Geometry check sheet. Reference: the model listing, model coordinates, mm. A direction names the side the tool comes from. Give positions to 0.01 mm unless a question says otherwise; leave off trailing zeros. Loops run counter-clockwise (first coordinate to the right, second up) from the corner with the lowest first, then second, coordinate; pieces in that order, holes last.
1. Go/stop test with flat-tipped pins: pin 1 Ø14 at (x, y) = (-53, 89.5) entering from -Z; pin 2 Ø1.2 at (y, z) = (77.5, 21) entering from +X. Record where each tip stops, or that it passes through.
2. Tool access check on faces 1 (the flat face through (-48, 0, 16)), 2 (the flat face through (-27, 63, 22.479)), 3 (the flat face through (-59, 63, 5.033)). Record the directions out of +Z, -Z, +X, -X, +Y, -Y that give a thin tool (end or side, any length) a straight path to the whole face; none if there is none.
3. Cross-section at B-B, the plane y = 29.5. Record the cut outline in (x, z), plus the area to 3 significant figures.
4. Cross-section at A-A, the plane z = 10.75. Record the cut outline in (x, y), plus the area to 3 significant figures.
5. Cross-section at C-C, the plane x = 28. Record the cut outline in (y, z), plus the area to 3 significant figures.
6. Cross-section at D-D, the plane x = 4. Record the cut outline in (y, z), plus the area to 3 significant figures.
7. Material ranges on L1, parallel to Z at x = 23, y = 116; L2, parallel to Y at x = -45, z = 20.5; L3, parallel to X at y = -40.5, z = 11.75, recorded low to high.
from build123d import *

# Parameters (mm, degrees)
F1_W     = 82.0750407875
F1_H     = 20.1075039804
F2_DEPTH = 50.7999993861
F0_W     = 82.0750407875
F0_H     = 20.1075039804
F4_DEPTH = 127


with BuildPart() as f2:
    # F1 (on face) → F2 (new body)
    with BuildSketch(Plane.XZ):
        with Locations((-3.4862887114, 10.0537519902)):
            Rectangle(F1_W, F1_H)
    extrude(amount=F2_DEPTH)

    # F3 (on face) + F0 (on Front) → F4 (join)
    with BuildSketch(Plane.XZ):
        Polygon((-72.149567306, 5.0325542688), (-44.5238091052, 5.0325542688), (-44.5238091052, 20.1075039804), (15.9993991256, 20.1075039804), (15.9993991256, 22.4787890911), (-72.149567306, 22.4787890911), align=None)
    with BuildSketch(Plane.XZ):
        with Locations((-3.4862887114, 10.0537519902)):
            Rectangle(F0_W, F0_H)
    extrude(amount=-F4_DEPTH)


solid = f2.part
Result:
1. pin 1: stops at z = 5.03
1. pin 2: stops at x = 16
2. face 1: +Z, -X, -Y
2. face 2: +Z, +X, -X, +Y, -Y
2. face 3: -Z, -X, +Y, -Y
3. outline: (-72.15, 5.03) - (-44.52, 5.03) - (-44.52, 0) - (37.55, 0) - (37.55, 20.11) - (16, 20.11) - (16, 22.48) - (-72.15, 22.48) - close
3. area: 2,280 mm2
4. outline: (-72.15, 0) - (-44.52, 0) - (-44.52, -50.8) - (37.55, -50.8) - (37.55, 127) - (-72.15, 127) - close
4. area: 18,100 mm2
5. outline: (-50.8, 0) - (127, 0) - (127, 20.11) - (-50.8, 20.11) - close
5. area: 3,580 mm2
6. outline: (-50.8, 0) - (127, 0) - (127, 22.48) - (0, 22.48) - (0, 20.11) - (-50.8, 20.11) - close
6. area: 3,880 mm2
7. L1: z = 0 to 20.11
7. L2: y = 0 to 127
7. L3: x = -44.52 to 37.55
